Build history of the part. All positions in model axes, mm. A direction names the side the tool comes from. Round coordinates to 2 decimals unless told otherwise and drop trailing zeros. Loops run counter-clockwise (first coordinate to the right, second up) from the corner with the lowest first, then second, coordinate; pieces in that order, holes last. Notation, with made-up numbers: (-23, 15.25) - (5, 15.25) arc R34 ccw to (5, 51.25) - close; hole circle Ø3 at (67.5, -28.75). An arc over 180 degrees is marked (long way). Use a Markdown table: item, result.
from build123d import *

# Parameters (mm, degrees)
SKETCH1_R          = 10
EXTRUDE1_DEPTH     = 15
EXTRUDE2_START     = 7
SKETCH2_R          = 10
EXTRUDE2_DEPTH     = 7
EXTRUDE5_DEPTH     = 33
SKETCH6_W          = 21.871062772
SKETCH6_H          = 26.824754441
CUT_EXTRUDE1_DEPTH = 101.943790616
SKETCH7_R          = 3.531045805
SKETCH7_R_2        = 3.594142414
CUT_EXTRUDE2_DEPTH = 81.795684194
FILLET6_R          = 5
SKETCH8_R          = 10.980976462
CUT_EXTRUDE3_DEPTH = 79.017105375


with BuildPart() as part:
    # Sketch1 → Extrude1 (new body)
    with BuildSketch(Plane.XY):
        with Locations((2, -17.227058485)):
            Circle(SKETCH1_R)
    extrude(amount=EXTRUDE1_DEPTH)

    # Sketch2 → Extrude2 (add)
    with BuildSketch(Plane(origin=(0, 0, 0), x_dir=(-1, 0, 0), z_dir=(0, 0, -1)).offset(EXTRUDE2_START)):
        with Locations((-2, -17.227058485)):
            Circle(SKETCH2_R)
    extrude(amount=-EXTRUDE2_DEPTH)

    # Sketch5 → Extrude5 (add)
    with BuildSketch(Plane(origin=(0, 0, 0), x_dir=(1, 0, 0), z_dir=(0, 1, 0))):
        Polygon((-15.907949581, 7), (-23.26436451, 17.67616864), (-23.26436451, 29.651727827), (-5.884555097, 29.651727827), (2.510054524, 19.69092733), (43.11444927, 19.69092733), (49.273308281, 30.678204329), (63.301820472, 30.678204329), (67.065567645, 19.69092733), (59.951736606, 7), align=None)
    extrude(amount=-EXTRUDE5_DEPTH)

    # Sketch6 → Cut-Extrude1 (cut, through all)
    with BuildSketch(Plane.ZY.offset(23.26436451)):
        with Locations((-21.908176834, -16.872312291)):
            Rectangle(SKETCH6_W, SKETCH6_H)
    extrude(amount=-CUT_EXTRUDE1_DEPTH, mode=Mode.SUBTRACT)

    # Sketch7 → Cut-Extrude2 (cut, through all)
    with BuildSketch(Plane(origin=(0, 0, 0), x_dir=(-1, 0, 0), z_dir=(0, 1, 0))):
        with Locations(Location((12.963937966, -22.243817104, 0), (0, 0, 90))):
            Circle(SKETCH7_R)
        with Locations(Location((-56.470516278, -22.243817104, 0), (0, 0, 90))):
            Circle(SKETCH7_R_2)
    extrude(amount=-CUT_EXTRUDE2_DEPTH, mode=Mode.SUBTRACT)

    # Fillet6
    fillet6_edges = [part.edges().sort_by_distance(p)[0] for p in [
        (-23.26436451, -31.642344755, -17.67616864),
        (-23.26436451, -31.642344755, -29.651727827),
        (-5.884555097, -31.642344755, -29.651727827),
        (2.510054524, -31.642344755, -19.69092733),
        (43.11444927, -31.642344755, -19.69092733),
        (49.273308281, -31.642344755, -30.678204329),
        (63.301820472, -31.642344755, -30.678204329),
        (67.065567645, -31.642344755, -19.69092733),
        (67.065567645, -1.729967535, -19.69092733),
        (63.301820472, -1.729967535, -30.678204329),
        (43.11444927, -1.729967535, -19.69092733),
        (2.510054524, -1.729967535, -19.69092733),
        (-5.884555097, -1.729967535, -29.651727827),
        (-23.26436451, -1.729967535, -29.651727827),
        (-23.26436451, -1.729967535, -17.67616864),
    ]]
    fillet(fillet6_edges, radius=FILLET6_R)

    # Sketch8 → Cut-Extrude3 (cut, through all)
    with BuildSketch(Plane.XY.offset(-7)):
        with Locations((34.285400433, -15.652526202)):
            Circle(SKETCH8_R)
    extrude(amount=-CUT_EXTRUDE3_DEPTH, mode=Mode.SUBTRACT)


solid = part.part
Q1. Which spindle directions (+Z, -Z, +X, -X, +Y, -Y) get a long thin tool onto all of the face, cutting with end or side? Do faces 4 (the face through (22, -2, -19.691)), 5 (the face through (-13, -2, -29.652)), 6 (the face through (49.64, -31.66, -29.97)), 7 (the face through (56, -32, -30.678)), 8 (the face through (21, -3.46, -19)). Say none if no direction does.
Results found:
| item | result |
|---|---|
| face 4 | -Z, +Y, -Y |
| face 5 | -Z, -X, +Y, -Y |
| face 6 | -Z, -Y |
| face 7 | -Z, +X, -X, +Y, -Y |
| face 8 | -Z, +X, -X |
Q2. Cut at A-A, the plane y = -19. List the corners of the cut face in (x, z), plus the area to 3 significant figures.
Results found:
| item | result |
|---|---|
| outline | (-18.65, -10.97) - (23.83, -10.97) - (23.83, -7) - (11.84, -7) - (11.84, 15) - (-7.84, 15) - (-7.84, -7) - (-15.91, -7) - close; (44.74, -10.97) - (62.18, -10.97) - (59.95, -7) - (44.74, -7) - close |
| area | 661 mm2 |
Q3. Drop flat-ended pins along their axis: pin 1 (2 mm diameter, centred on x = 15.5, y = -32, fed in from -Z); pin 2 (9 mm diameter, centred on x = -12.96, z = -22.24, fed in from +Y); pin 3 (3 mm diameter, centred on x = -13.5, y = -1, fed in from -Z); pin 4 (4 mm diameter, centred on x = -5.5, y = -29, fed in from -Z). Give the stop position or say it passes through.
Results found:
| item | result |
|---|---|
| pin 1 | stops at z = -19.69 |
| pin 2 | stops at y = 0 |
| pin 3 | stops at z = -29.65 |
| pin 4 | stops at z = -29.51 |
Q4. Cut at B-B, the plane x = 34.5. List the corners of the cut face in (y, z), plus the area to 3 significant figures.
Results found:
| item | result |
|---|---|
| outline | (-33, -19.69) - (-30.28, -19.69) - (-30.28, -10.97) - (-26.63, -10.97) - (-26.63, -7) - (-33, -7) - close; (-4.67, -10.97) - (-3.46, -10.97) - (-3.46, -19.69) - (0, -19.69) - (0, -7) - (-4.67, -7) - close |
| area | 97.7 mm2 |
Q5. Cut at C-C, the plane x = -10.5. List the corners of the cut face in (y, z), plus the area to 3 significant figures.
Results found:
| item | result |
|---|---|
| outline | (-33, -29.65) - (-30.28, -29.65) - (-30.28, -24.77) - (-33, -24.77) - close; (-33, -19.71) - (-30.28, -19.71) - (-30.28, -10.97) - (-3.46, -10.97) - (-3.46, -19.71) - (0, -19.71) - (0, -7) - (-33, -7) - close; (-3.46, -29.65) - (0, -29.65) - (0, -24.77) - (-3.46, -24.77) - close |
| area | 215 mm2 |
Q6. Probe line 1 (Z direction, x = -10.5, y = -11); line 2 (Z direction, x = 31, y = -2); line 3 (Y direction, x = 13, z = -15.5). List the from-to ranges inside material, lowest first.
Results found:
| item | result |
|---|---|
| line 1 | z = -10.97 to -7 |
| line 2 | z = -19.69 to -7 |
| line 3 | y = -33 to -30.28, -3.46 to 0 |
Q7. Pull direction Y, two halves, no side cores. Call faces 1 (the face through (22, -33, -16)), 2 (the face through (-6.13, -1.75, -29.2)), 3 (the face through (23.315, -15.17, -8.959)): pulls with the +Y half, pulls with the -Y half, needs draft (parallel to the pull), parting line crosses it, or undercut.
Results found:
| item | result |
|---|---|
| face 1 | pulls with the -Y half |
| face 2 | needs draft |
| face 3 | undercut |
Q8. Cut at D-D, the plane z = -9. List the corners of the cut face in (x, y), plus the area to 3 significant figures.
Results found:
| item | result |
|---|---|
| outline | (-17.29, -33) - (61.07, -33) - (61.07, 0) - (-17.29, 0) - close; hole circle Ø21.96 at (34.29, -15.65) |
| area | 2,210 mm2 |
